Could you check a few things on this model? Use its own coordinates, in mm. A direction names the side the tool comes from. Give positions to 0.01 mm unless a question says otherwise; leave off trailing zeros. Order: outer loops, then holes, each group sorted by start corner. A loop starts at its lowest first (then second) coordinate and runs counter-clockwise, first axis right, second up. Notation, with made-up numbers: (-22.75, -18) - (-17.75, -18) arc R18 ccw to (-17.75, -1) - close; hole circle Ø8 at (62, 5). An arc over 180 degrees is marked (long way). Put each result on its own line as item: value.
from build123d import *

# Parameters (mm, degrees)
F1_DEPTH    = 3
F3_DEPTH    = 3
F5_DEPTH    = 2
F7_DEPTH    = 2
F8_W        = 3
F8_H        = 30
F9_DEPTH    = 1
F10_SIZE2   = 2.99999
F10_SIZE    = 0.99999
F10_2_SIZE2 = 2.99999
F10_2_SIZE  = 0.99999


# Not quite as in the source:
# - a fillet or chamfer is up to 0.001 mm smaller than in the source, because OpenCascade refuses the exact size


with BuildPart() as f1:
    # F0 (on Top) → F1 (new body)
    with BuildSketch(Plane.XY):
        with BuildLine():
            ThreePointArc((0, -56), (4.4433524368, -28), (0, 0))
            Line((0, 0), (-46, 0))
            ThreePointArc((-46, 0), (-50.4433524368, -28), (-46, -56))
            Line((-46, -56), (0, -56))
        make_face()
    extrude(amount=F1_DEPTH)

    # F2 (on face) → F3 (join)
    with BuildSketch(Plane.XY.offset(3)):
        Polygon((-38, -13), (-41, -13), (-41, -43), (-38, -43), (-38, -40.5), (-36, -40.5), (-36, -15.5), (-38, -15.5), align=None)
        Polygon((-5, -43), (-5, -13), (-8, -13), (-8, -15.5), (-10, -15.5), (-10, -40.5), (-8, -40.5), (-8, -43), align=None)
    extrude(amount=F3_DEPTH)

    # F4 (on face) → F5 (join)
    with BuildSketch(Plane.XY.offset(6)):
        Polygon((-38, -13), (-41, -13), (-41, -43), (-38, -43), (-38, -40.5), (-36, -40.5), (-32.5, -37.5), (-32.5, -18.5), (-36, -15.5), (-38, -15.5), align=None)
    extrude(amount=F5_DEPTH)

    # F6 (on face) → F7 (join)
    with BuildSketch(Plane.XY.offset(6)):
        Polygon((-5, -13), (-8, -13), (-8, -15.5), (-10, -15.5), (-13.5, -18.5), (-13.5, -37.5), (-10, -40.5), (-8, -40.5), (-8, -43), (-5, -43), align=None)
    extrude(amount=F7_DEPTH)

    # F8 (on face) → F9 (join)
    with BuildSketch(Plane.XY.offset(3)):
        with Locations((-23, -28)):
            Rectangle(F8_W, F8_H)
    extrude(amount=F9_DEPTH)

    # F10 (size 1 and 3 in the source; OpenCascade refuses exactly that, so slightly less here)
    f10_edges = [f1.edges().sort_by_distance(p)[0] for p in [
        (-23, -13, 4),
    ]]
    f10_side = f1.faces().sort_by_distance((-23, -13, 3.5))[0]
    chamfer(f10_edges, length=F10_SIZE, length2=F10_SIZE2, reference=f10_side)

    # F10#2 (size 1 and 3 in the source; OpenCascade refuses exactly that, so slightly less here)
    f10_2_edges = [f1.edges().sort_by_distance(p)[0] for p in [
        (-23, -43, 4),
    ]]
    f10_2_side = f1.faces().sort_by_distance((-23, -43, 3.5))[0]
    chamfer(f10_2_edges, length=F10_2_SIZE, length2=F10_2_SIZE2, reference=f10_2_side)


solid = f1.part
1) Suppose I cut it at A-A, the plane x = -7. List the corners of the cut face in (y, z) for me.
Filled in:
outline: (-56, 0) - (0, 0) - (0, 3) - (-13, 3) - (-13, 8) - (-43, 8) - (-43, 3) - (-56, 3) - close
2) We'd pull the mould along X, two halves only. Please class faces 5 (the flat face through (-39, -13, 5)), 6 (the flat face through (-36, -28, 4)), 7 (the cylindrical face through (4.442, -28.399, 1.479)): pulls with the +X half, pulls with the -X half, needs draft (parallel to the pull), parting line crosses it, or undercut.
Filled in:
face 5: needs draft
face 6: undercut
face 7: pulls with the +X half
3) Suppose I cut it at C-C, the plane y = -31. List the corners of the cut face in (x, z) for me, and give its area (3 significant figures).
Filled in:
outline: (-50.39, 0) - (4.39, 0) - (4.39, 3) - (-5, 3) - (-5, 8) - (-13.5, 8) - (-13.5, 6) - (-10, 6) - (-10, 3) - (-21.5, 3) - (-21.5, 4) - (-24.5, 4) - (-24.5, 3) - (-36, 3) - (-36, 6) - (-32.5, 6) - (-32.5, 8) - (-41, 8) - (-41, 3) - (-50.39, 3) - close
area: 231 mm^2
4) If I drill on line 1 (Z direction, x = -12, y = -29); line 2 (X direction, y = -13.5, z = 3.75); line 3 (X direction, y = -25, z = 5.5), over which ranges is the centre line in solid material (lowest first)? Write a range as [from, to].
Filled in:
line 1: z = [0, 3], [6, 8]
line 2: x = [-41, -38], [-8, -5]
line 3: x = [-41, -36], [-10, -5]
5) Suppose I cut it at D-D, the plane y = -17. List the corners of the cut face in (x, z) for me.
Filled in:
outline: (-49.77, 0) - (3.77, 0) - (3.77, 3) - (-5, 3) - (-5, 8) - (-11.75, 8) - (-11.75, 6) - (-10, 6) - (-10, 3) - (-21.5, 3) - (-21.5, 4) - (-24.5, 4) - (-24.5, 3) - (-36, 3) - (-36, 6) - (-34.25, 6) - (-34.25, 8) - (-41, 8) - (-41, 3) - (-49.77, 3) - close
6) Which directions (+Z, -Z, +X, -X, +Y, -Y) give clear straight access to the entire face, cutting with the end or side of a thin tool? Please do faces 1 (the flat face through (-23, -28, 4)), 2 (the flat face through (-12, -28, 6)), 3 (the flat face through (-9, -40.5, 5)), 4 (the flat face through (-41, -28, 5)).
Filled in:
face 1: +Z, +Y, -Y
face 2: +Y, -Y
face 3: +Z, -Y
face 4: +Z, -X, +Y, -Y
7) Suppose I cut it at B-B, the plane y = -5. List the corners of the cut face in (x, z) for me.
Filled in:
outline: (-47.47, 0) - (1.47, 0) - (1.47, 3) - (-47.47, 3) - close
8) I'm going to push flat-ended pins straight in: pin 1 (2.5 mm diameter, centred on y = -33.5, z = 6.5, fed in from +X); pin 2 (1.1 mm diameter, centred on y = -29.5, z = 3.5, fed in from +X); pin 3 (0.9 mm diameter, centred on x = -7, z = 4.5, fed in from -Y). Where does each tip first touch, or does it pass through?
Filled in:
pin 1: stops at x = -5
pin 2: stops at x = 4.43
pin 3: stops at y = -43
